Source: three-view drawing plus pictorial views. Frame: mm from the lowest corner of the part. A direction names the side the tool comes from. Round coordinates to 2 decimals unless told otherwise and drop trailing zeros. Loops run counter-clockwise (first coordinate to the right, second up) from the corner with the lowest first, then second, coordinate; pieces in that order, holes last. Notation, with made-up numbers: (11.5, 73.5) -> (53.5, 73.5) arc R23 ccw to (53.5, 81.5) -> close; hole circle Ø1 at (-32.75, 88.5). An arc over 180 degrees is marked (long way). Answer in a Markdown table with one row per item.
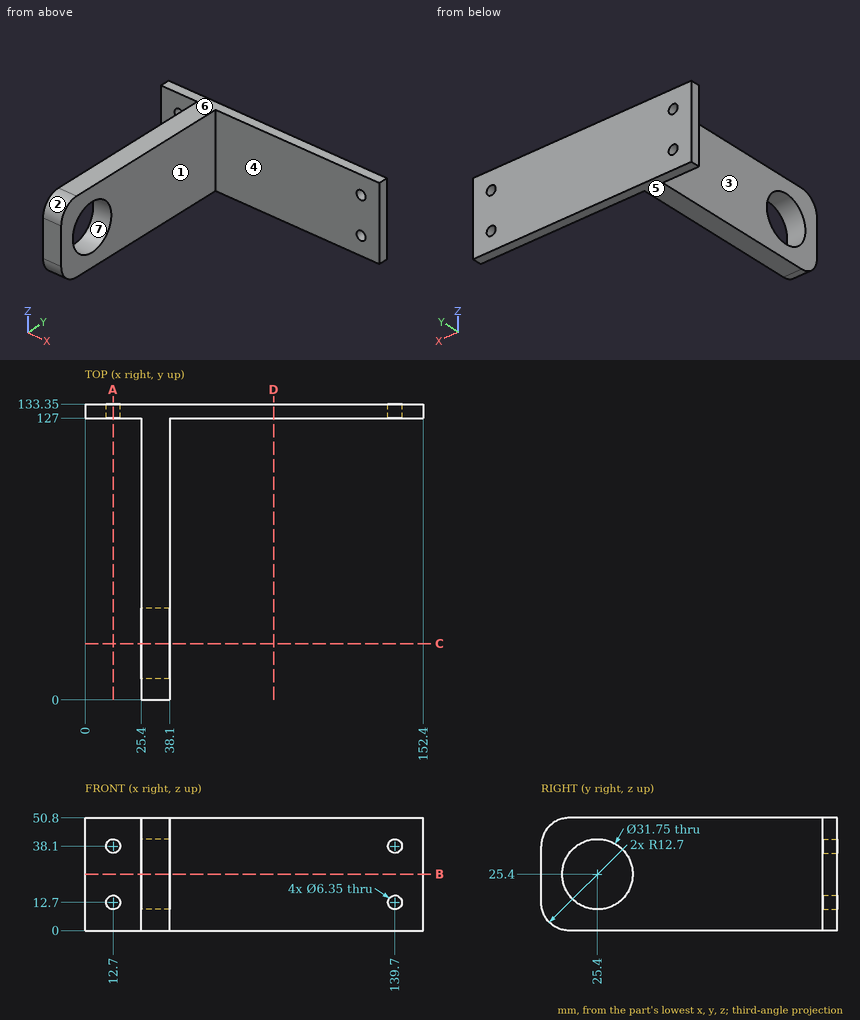
Item 1: Reachability of the marked faces 1, 2 and 3 from +Z, -Z, +X, -X, +Y, -Y: full face, straight path, thin tool, end or side. Return the list, or none.
Answer:
| item | result |
|---|---|
| face 1 | +Z, -Z, +X, -Y |
| face 2 | +Z, +X, -X, -Y |
| face 3 | +Z, -Z, -X, -Y |
Item 2: Cut plane C-C (y = 25.4). Output: boundary loops of the cut face in (x, z) (3 decimals), then the cut area to 3 significant figures.
Answer:
| item | result |
|---|---|
| outline | (25.4, 0) -> (38.1, 0) -> (38.1, 9.525) -> (25.4, 9.525) -> close; (25.4, 41.275) -> (38.1, 41.275) -> (38.1, 50.8) -> (25.4, 50.8) -> close |
| area | 242 mm² |
Item 3: Pin query (flat end, axial travel): pin 1 Ø12 at (y, z) = (75.5, 19.5) entering from -X; pin 2 Ø10 at (x, z) = (139.7, 38.1) entering from -Y; pin 3 Ø6 at (y, z) = (77.5, 31.5) entering from +X. Return the tip coordinate at first contact, or that it passes through.
Answer:
| item | result |
|---|---|
| pin 1 | stops at x = 25.4 |
| pin 2 | stops at y = 127 |
| pin 3 | stops at x = 38.1 |
Item 4: Line query: probe 1 along Z at (x, y) = (139.7, 130.25) (3 decimals); probe 2 along Z at (x, y) = (32.75, 25.4) (3 decimals); probe 3 along X at (y, z) = (110.5, 21). Output: solid intervals per line, ascending. Write a range as [from, to].
Answer:
| item | result |
|---|---|
| probe 1 | z = [0, 9.525], [15.875, 34.925], [41.275, 50.8] |
| probe 2 | z = [0, 9.525], [41.275, 50.8] |
| probe 3 | x = [25.4, 38.1] |
Item 5: Cut plane A-A (x = 12.7). Output: boundary loops of the cut face in (y, z) (3 decimals).
Answer:
| item | result |
|---|---|
| outline | (127, 0) -> (133.35, 0) -> (133.35, 9.525) -> (127, 9.525) -> close; (127, 15.875) -> (133.35, 15.875) -> (133.35, 34.925) -> (127, 34.925) -> close; (127, 41.275) -> (133.35, 41.275) -> (133.35, 50.8) -> (127, 50.8) -> close |
Item 6: Cut plane D-D (x = 85). Output: boundary loops of the cut face in (y, z), then the cut area to 3 significant figures.
Answer:
| item | result |
|---|---|
| outline | (127, 0) -> (133.35, 0) -> (133.35, 50.8) -> (127, 50.8) -> close |
| area | 323 mm² |
Item 7: Draft query along Z for the marked faces 4, 5, 6 and 7. Return one class per face: pulls with the +Z half, pulls with the -Z half, needs draft (parallel to the pull), parting line crosses it, or undercut.
Answer:
| item | result |
|---|---|
| face 4 | needs draft |
| face 5 | pulls with the -Z half |
| face 6 | pulls with the +Z half |
| face 7 | undercut |
Item 8: Cut plane B-B (z = 25.4). Output: boundary loops of the cut face in (x, y) (3 decimals), then the cut area to 3 significant figures.
Answer:
| item | result |
|---|---|
| outline | (0, 127) -> (25.4, 127) -> (25.4, 41.275) -> (38.1, 41.275) -> (38.1, 127) -> (152.4, 127) -> (152.4, 133.35) -> (0, 133.35) -> close; (25.4, 0) -> (38.1, 0) -> (38.1, 9.525) -> (25.4, 9.525) -> close |
| area | 2,180 mm² |
